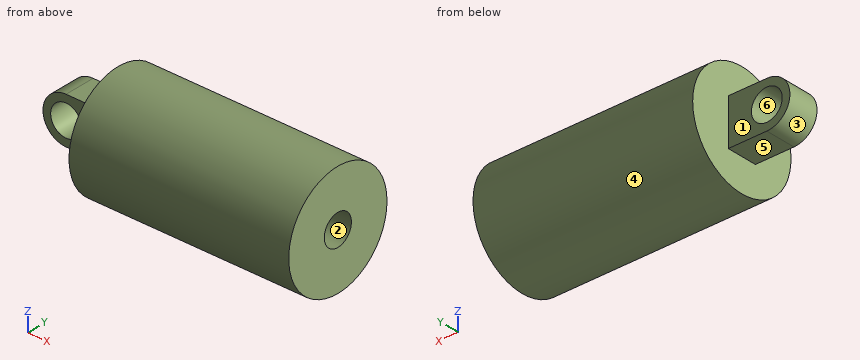
Autodesk Inventor part; units mm, degrees
ref_plane "YZ Plane" through (0, 0, 0) normal (1, 0, 0) x (0, 1, 0)
ref_plane "XZ Plane" through (0, 0, 0) normal (0, 1, 0) x (-1, 0, 0)
ref_plane "XY Plane" through (0, 0, 0) normal (0, 0, 1) x (1, 0, 0)
sketch "スケッチ1" plane through (0, 0, 0) normal (1, 0, 0) x (0, 1, 0)
  circle A0 centre (0, 0) radius 7.25
  dimension "d0" = 14.5
extrude "押し出し1" add sketch "スケッチ1" along normal blind 28.5
sketch "スケッチ2" plane through (0, 0, 0) normal (0, 1, 0) x (-1, 0, 0)
  circle A0 centre (5, 0) radius 2
  circle A1 centre (5, 0) radius 3
  line L0 (5, -3) -> (0, -3)
  line L1 (0, 7.25) -> (0, -7.25)
  line L2 (5, 3) -> (0, 3)
  point P0 (0, 0)
  dimension "d3" = 4
  dimension "d4" = 5
  dimension "d5" = 6
extrude "押し出し2" add sketch "スケッチ2" along normal mid plane 4
sketch "スケッチ3" plane through (28.5, 0, 0) normal (1, 0, 0) x (0, 0, -1)
  circle A0 centre (0, 0) radius 2
  dimension "d8" = 4
extrude "押し出し3" cut sketch "スケッチ3" against normal blind 10
properties part number "pink-suspension-under" material "ABS プラスチック"
For this review, take the finished solid that the model builds, in its own axes (mm). Face numbers are marked on the shaded views. A direction names the side the tool comes from. Give positions to 0.01 mm unless a question says otherwise; leave off trailing zeros. Loops run counter-clockwise (first coordinate to the right, second up) from the corner with the lowest first, then second, coordinate; pieces in that order, holes last. Notation, with made-up numbers: (6.5, -39.5) - (40.5, -39.5) arc R28 ccw to (40.5, -14.5) - close; hole circle Ø2 at (86, 27.25). An arc over 180 degrees is marked (long way). Write each question's results on one line, items separated by ' | '.
(1) For the marked faces 5 and 6, list the 3-axis set-ups (+Z, -Z, +X, -X, +Y, -Y) from which the entire face can be reached by the end or side of a thin tool; tool diameter is ignored.
Conclusion:
face 5: -Z, -X, +Y, -Y | face 6: +Y, -Y
(2) For pin 1 Ø3 at (x, z) = (24, -4) entering from -Y; pin 2 Ø2 at (y, z) = (-4, -0.5) entering from -X; pin 3 Ø1.8 at (x, z) = (-2.5, 0.5) entering from +Y; pin 4 Ø6.5 at (x, z) = (-3, 0) entering from -Y, all flat-tipped, find the tip position at first contact; note any pin that passes through.
Conclusion:
pin 1: y = -6.81 | pin 2: x = 0 | pin 3: y = 2 | pin 4: y = -7.25
(3) Take a section at A-A (y = 0). Give the boundary of the cut face in (x, z), then the cut area to 3 significant figures.
Conclusion:
outline: (-5, -3) - (0, -3) - (0, -7.25) - (28.5, -7.25) - (28.5, -2) - (18.5, -2) - (18.5, 2) - (28.5, 2) - (28.5, 7.25) - (0, 7.25) - (0, 3) - (-5, 3) arc R3 ccw to start; hole circle Ø4 at (-5, 0) | area: 405 mm^2
(4) Draft analysis for pull direction Y (two halves, no side actions). For the marked faces 1, 2, 3 and 4, state which applies: +Y half, -Y half, draft (parallel to the pull), parting line (faces both ways), or undercut.
Conclusion:
face 1: +Y half | face 2: undercut | face 3: draft | face 4: parting line
(5) Take a section at C-C (x = 24). Give the boundary of the cut face in (y, z).
Conclusion:
outline: circle Ø14.5 at (0, 0); hole circle Ø4 at (0, 0)
(6) Take a section at B-B (z = -1.5). Give the boundary of the cut face in (x, y), then the cut area to 3 significant figures.
Conclusion:
outline: (-7.6, -2) - (-6.32, -2) - (-6.32, 2) - (-7.6, 2) - close; (-3.68, -2) - (0, -2) - (0, -7.09) - (28.5, -7.09) - (28.5, -1.32) - (18.5, -1.32) - (18.5, 1.32) - (28.5, 1.32) - (28.5, 7.09) - (0, 7.09) - (0, 2) - (-3.68, 2) - close | area: 398 mm^2
(7) Take a section at D-D (z = 0). Give the boundary of the cut face in (x, y).
Conclusion:
outline: (-8, -2) - (-7, -2) - (-7, 2) - (-8, 2) - close; (-3, -2) - (0, -2) - (0, -7.25) - (28.5, -7.25) - (28.5, -2) - (18.5, -2) - (18.5, 2) - (28.5, 2) - (28.5, 7.25) - (0, 7.25) - (0, 2) - (-3, 2) - close
(8) For line 1 along Z through (x, y) = (-5, 0.8); line 2 along X through (y, z) = (2.5, 3.25); line 3 along Y through (x, z) = (5, 0.25), list the stretches that pass through material, from the lowest coordinate up.
Conclusion:
line 1: -3 to -2, 2 to 3 | line 2: 0 to 28.5 | line 3: -7.25 to 7.25
